Geometry check sheet. Reference: the model listing, model coordinates, mm. A direction names the side the tool comes from. Coordinates: 2 decimals unless noted, no trailing zeros. Write each loop counter-clockwise with the first axis right and the second up, starting at its lowest first coordinate (ties: lowest second). Pieces come first, ordered by that corner, then holes. Notation, with made-up numbers: M 81,-35.5 L 124,-35.5 A23 ccw 124,-2.5 Z; hole C 5,-30 d2. An arc over 180 degrees is marked long. Put each result on its own line as item: value. Start each with the question number.
1) Cross-section at B-B on y = 33.5. Record the cut outline in (x, z).
2) Cross-section at A-A on x = -37.5. Record the cut outline in (y, z), plus the area to 3 significant figures.
3) Scan lines: line 1 along Z through (x, y) = (-20.5, 55.5); line 2 along Y through (x, z) = (-18.5, 22.5); line 3 along X through (y, z) = (20.5, 3.5). Record each from-to range of solid material in increasing order.
4) Cross-section at D-D on y = 53.5. Record the cut outline in (x, z).
5) Cross-section at C-C on z = 6.5. Record the cut outline in (x, y).
6) Set-up check for faces 1 (the cylindrical face through (-28.175, 40.866, 12.522)), 2 (the flat face through (-26, 0, -6)): record each of +Z, -Z, +X, -X, +Y, -Y from which the full face is reachable in a straight line by a thin tool's end or side.
7) Gauge pin test, flat ends, axial feed: pin 1 (1 mm diameter, centred on y = 38.5, z = 3, fed in from -X); pin 2 (12 mm diameter, centred on x = -25, z = 21.5, fed in from +Y); pin 3 (1.5 mm diameter, centred on y = 38.5, z = 15, fed in from -X). Record the tip position at first contact, or that the pin passes through.
from build123d import *

# Parameters (mm, degrees)
F0_W     = 38.70645
F0_H     = 57.275925
F1_DEPTH = 12.7
F2_R     = 12.174497
F3_DEPTH = 25.4


with BuildPart() as f1:
    # F0 (on Top) → F1 (new body)
    with BuildSketch(Plane.XY):
        with Locations((-25.682018, 28.637963)):
            Rectangle(F0_W, F0_H)
    extrude(amount=-F1_DEPTH)

    # F2 (on face) → F3 (join)
    with BuildSketch(Plane.XY):
        with Locations((-26.59025, 28.795289)):
            Circle(F2_R)
    extrude(amount=F3_DEPTH)


solid = f1.part
Answer key:
1. outline: M -45.04,-12.7 L -6.33,-12.7 L -6.33,0 L -15.36,0 L -15.36,25.4 L -37.82,25.4 L -37.82,0 L -45.04,0 Z
2. outline: M 0,-12.7 L 57.28,-12.7 L 57.28,0 L 34.2,0 L 34.2,25.4 L 23.39,25.4 L 23.39,0 L 0,0 Z
2. area: 1,000 mm²
3. line 1: z = -12.7 to 0
3. line 2: y = 19.7 to 37.89
3. line 3: x = -35.5 to -17.68
4. outline: M -45.04,-12.7 L -6.33,-12.7 L -6.33,0 L -45.04,0 Z
5. outline: C -26.59,28.8 d24.35
6. face 1: +Z
6. face 2: +Z, -Z, +X, -X, -Y
7. pin 1: stops at x = -34.56
7. pin 2: stops at y = 40.97
7. pin 3: stops at x = -34.84
